Autodesk Inventor part; units mm, degrees
ref_plane "YZ Plane" through (0, 0, 0) normal (1, 0, 0) x (0, 1, 0)
ref_plane "XZ Plane" through (0, 0, 0) normal (0, 1, 0) x (-1, 0, 0)
ref_plane "XY Plane" through (0, 0, 0) normal (0, 0, 1) x (1, 0, 0)
sketch "Skizze1" plane through (0, 0, 0) normal (0, 0, 1) x (1, 0, 0)
  line L0 (25, 12.5) -> (-25, 12.5)
  line L1 (-25, 12.5) -> (-25, -12.5)
  line L2 (-25, -12.5) -> (25, -12.5)
  line L3 (25, -12.5) -> (25, 12.5)
  circle A0 centre (50.8, -8.2735) radius 14.6905
  circle A1 centre (50.8, -8.2735) radius 15
  line L4 (-63.7896, 27.9801) -> (95.321, 27.9801)
  line L5 (95.321, 27.9801) -> (95.321, -42.1521)
  line L6 (95.321, -42.1521) -> (-63.7896, -42.1521)
  line L7 (-63.7896, -42.1521) -> (-63.7896, 27.9801)
  point P0 (0, 0)
  dimension "d0" = 30
extrude "Extrusion1" add sketch "Skizze1" along normal blind 3 contours L4 L5 L6 L7
sketch "Skizze2" plane through (0, 0, 0) normal (0, 0, -1) x (-1, 0, 0)
  circle A0 centre (-50.8, -8.2735) radius 15 construction
  circle A1 centre (-50.8, -8.2735) radius 17.5
  point P0 (0, 0)
  dimension "d3" = 35
extrude "Extrusion2" cut sketch "Skizze2" against normal blind 1
sketch "Skizze3" plane through (0, 0, 0) normal (0, 0, -1) x (-1, 0, 0)
  circle A0 centre (-77.33, -20.3235) radius 1.75 construction
  circle A1 centre (40.52, -20.3235) radius 1.75 construction
  circle A2 centre (40.52, 8.5265) radius 1.75 construction
  circle A3 centre (-77.33, 8.5265) radius 1.75 construction
  arc A4 (-44.8513, -25.2196) -> (-44.1338, -24.9216) centre (-45.6338, -22.3235) ccw construction
  arc A5 (-44.8513, -25.2196) -> (-45.0539, -25.3294) centre (-44.7209, -25.7023) ccw construction
  arc A6 (-46.2827, -25.4102) -> (-45.0539, -25.3294) centre (-45.72, -24.5835) ccw construction
  arc A7 (-46.2827, -25.4102) -> (-46.564, -25.3235) centre (-46.564, -25.8235) ccw construction
  line L0 (-55.036, -25.3235) -> (-46.564, -25.3235) construction
  arc A8 (-55.036, -25.3235) -> (-55.3173, -25.4102) centre (-55.036, -25.8235) ccw construction
  arc A9 (-56.4427, -25.4102) -> (-55.3173, -25.4102) centre (-55.88, -24.5835) ccw construction
  arc A10 (-56.4427, -25.4102) -> (-56.724, -25.3235) centre (-56.724, -25.8235) ccw construction
  line L1 (-66.83, -25.3235) -> (-56.724, -25.3235) construction
  arc A11 (-67.83, -24.3235) -> (-66.83, -25.3235) centre (-66.83, -24.3235) ccw construction
  line L2 (-67.83, -14.2262) -> (-67.83, -24.3235) construction
  arc A12 (-67.83, -14.2262) -> (-67.9233, -13.9353) centre (-68.33, -14.2262) ccw construction
  arc A13 (-67.9233, -12.7717) -> (-67.9233, -13.9353) centre (-67.11, -13.3535) ccw construction
  arc A14 (-67.9233, -12.7717) -> (-67.83, -12.4808) centre (-68.33, -12.4808) ccw construction
  line L3 (-67.83, -4.0662) -> (-67.83, -12.4808) construction
  arc A15 (-67.83, -4.0662) -> (-67.9233, -3.7753) centre (-68.33, -4.0662) ccw construction
  arc A16 (-67.9233, -2.6117) -> (-67.9233, -3.7753) centre (-67.11, -3.1935) ccw construction
  arc A17 (-67.9233, -2.6117) -> (-67.83, -2.3208) centre (-68.33, -2.3208) ccw construction
  line L4 (-67.83, -1.6101) -> (-67.83, -2.3208) construction
  arc A18 (-67.83, -1.6101) -> (-68.1376, -1.1483) centre (-68.3305, -1.6101) ccw construction
  arc A19 (-68.445, -0.6869) -> (-68.1376, -1.1483) centre (-67.945, -0.6869) ccw construction
  line L5 (-68.445, 14.5865) -> (-68.445, -0.6869) construction
  arc A20 (-67.945, 15.0865) -> (-68.445, 14.5865) centre (-67.945, 14.5865) ccw construction
  line L6 (-58.801, 15.0865) -> (-67.945, 15.0865) construction
  arc A21 (-58.301, 14.5865) -> (-58.801, 15.0865) centre (-58.801, 14.5865) ccw construction
  line L7 (-58.301, 14.5265) -> (-58.301, 14.5865) construction
  arc A22 (-58.301, 14.5265) -> (-57.301, 13.5265) centre (-57.301, 14.5265) ccw construction
  line L8 (-44.045, 13.5265) -> (-57.301, 13.5265) construction
  arc A23 (-44.045, 13.5265) -> (-43.045, 14.5265) centre (-44.045, 14.5265) ccw construction
  line L9 (-43.045, 14.5865) -> (-43.045, 14.5265) construction
  arc A24 (-42.545, 15.0865) -> (-43.045, 14.5865) centre (-42.545, 14.5865) ccw construction
  line L10 (-33.401, 15.0865) -> (-42.545, 15.0865) construction
  arc A25 (-32.901, 14.5865) -> (-33.401, 15.0865) centre (-33.401, 14.5865) ccw construction
  line L11 (-32.901, 14.5265) -> (-32.901, 14.5865) construction
  arc A26 (-32.901, 14.5265) -> (-31.901, 13.5265) centre (-31.901, 14.5265) ccw construction
  line L12 (21.02, 13.5265) -> (-31.901, 13.5265) construction
  arc A27 (31.02, 3.5265) -> (21.02, 13.5265) centre (21.02, 3.5265) ccw construction
  line L13 (31.02, 2.4539) -> (31.02, 3.5265) construction
  arc A28 (31.02, 2.4539) -> (31.3225, 1.9945) centre (31.52, 2.4539) ccw construction
  arc A29 (31.3225, -0.7615) -> (31.3225, 1.9945) centre (30.73, 0.6165) ccw construction
  arc A30 (31.3225, -0.7615) -> (31.02, -1.2209) centre (31.52, -1.2209) ccw construction
  line L14 (31.02, -1.3561) -> (31.02, -1.2209) construction
  arc A31 (31.02, -1.3561) -> (31.3225, -1.8155) centre (31.52, -1.3561) ccw construction
  arc A32 (31.3225, -4.5715) -> (31.3225, -1.8155) centre (30.73, -3.1935) ccw construction
  arc A33 (31.3225, -4.5715) -> (31.02, -5.0309) centre (31.52, -5.0309) ccw construction
  line L15 (31.02, -5.1661) -> (31.02, -5.0309) construction
  arc A34 (31.02, -5.1661) -> (31.3225, -5.6255) centre (31.52, -5.1661) ccw construction
  arc A35 (31.3225, -8.3815) -> (31.3225, -5.6255) centre (30.73, -7.0035) ccw construction
  arc A36 (31.3225, -8.3815) -> (31.02, -8.8409) centre (31.52, -8.8409) ccw construction
  line L16 (31.02, -10.4303) -> (31.02, -8.8409) construction
  arc A37 (31.02, -10.4303) -> (31.3433, -10.898) centre (31.52, -10.4303) ccw construction
  arc A38 (31.3433, -12.769) -> (31.3433, -10.898) centre (30.99, -11.8335) ccw construction
  arc A39 (31.3433, -12.769) -> (31.02, -13.2367) centre (31.52, -13.2367) ccw construction
  line L17 (31.02, -20.5903) -> (31.02, -13.2367) construction
  arc A40 (31.02, -20.5903) -> (31.3433, -21.058) centre (31.52, -20.5903) ccw construction
  arc A41 (31.3283, -22.9345) -> (31.3433, -21.058) centre (30.99, -21.9935) ccw construction
  arc A42 (31.3283, -22.9345) -> (30.9977, -23.3898) centre (31.4974, -23.4051) ccw construction
  arc A43 (28.77, -25.3235) -> (30.9977, -23.3898) centre (28.77, -23.0735) ccw construction
  line L18 (-24.9736, -25.3235) -> (28.77, -25.3235) construction
  arc A44 (-26.4736, -24.9216) -> (-24.9736, -25.3235) centre (-24.9736, -22.3235) ccw construction
  line L19 (-33.8037, -20.6895) -> (-26.4736, -24.9216) construction
  arc A45 (-33.8037, -20.6895) -> (-36.8037, -20.6895) centre (-35.3037, -23.2876) ccw construction
  line L20 (-44.1338, -24.9216) -> (-36.8037, -20.6895) construction
  line L21 (-81.83, -30.3235) -> (45.02, -30.3235) construction
  arc A46 (45.02, -30.3235) -> (48.02, -27.3235) centre (45.02, -27.3235) ccw construction
  line L22 (48.02, -27.3235) -> (48.02, 15.5265) construction
  arc A47 (48.02, 15.5265) -> (45.02, 18.5265) centre (45.02, 15.5265) ccw construction
  line L23 (45.02, 18.5265) -> (-81.83, 18.5265) construction
  arc A48 (-81.83, 18.5265) -> (-84.83, 15.5265) centre (-81.83, 15.5265) ccw construction
  line L24 (-84.83, 15.5265) -> (-84.83, -27.3235) construction
  arc A49 (-84.83, -27.3235) -> (-81.83, -30.3235) centre (-81.83, -27.3235) ccw construction
  point P0 (0, 0)
hole "Bohrung1" at (77.33, 8.5265, 0) at (77.33, -20.3235, 0) at (-40.52, -20.3235, 0) at (-40.52, 8.5265, 0) direction (0, 0, 1) diameter 3 end through all
properties part number "Ausschnitt"
CAD build for the part. Positions are in the model's coordinates, mm. A direction names the side the tool comes from. Coordinates: 2 decimals unless noted, no trailing zeros. Write each loop counter-clockwise with the first axis right and the second up, starting at its lowest first coordinate (ties: lowest second). Pieces come first, ordered by that corner, then holes. Notation, with made-up numbers: (-8, 11) - (10, 11) arc R23 ccw to (10, 21) - close; hole circle Ø7 at (79, 46.5). An arc over 180 degrees is marked (long way). Use a Markdown table: item, result. Add a question column.
Item 1: Band-saw the part on B-B, the plane y = -1.5. Give the cut face in (x, z).
Item 2: Drill centre lines: L1, parallel to Y at x = -40.52, z = 2.35; L2, parallel to Y at x = 50.8, z = 2.65; L3, parallel to X at y = -2, z = 1.6. Where is each one in solid material? Low to high. Write a range as from..to.
Item 3: Band-saw the part on C-C, the plane x = -40.52. Give the cut face in (y, z), and give its area (3 significant figures).
Item 4: Band-saw the part on D-D, the plane z = 1.9. Give the cut face in (x, y), and give its area (3 significant figures).
Item 5: Mould opens along Y. For faces 1 (the face through (78.794, -20.649, 1.521)), 2 (the face through (17, -42.152, 1)), 3 (the face through (-63.79, -8, 1)) say: pulls with the +Y half, pulls with the -Y half, needs draft (parallel to the pull), parting line crosses it, or undercut.
Item 6: 3-axis set-ups, long thin cutter, end or side, ignore diameter. For faces 4 (the face through (68.283, -7.504, 0.493)), 5 (the face through (0, 12.5, 1)), 6 (the face through (15, -14, 0)): which of +Z, -Z, +X, -X, +Y, -Y reach the whole face in a straight line?
Item 7: Band-saw the part on A-A, the plane x = 50.8. Give the cut face in (y, z), and give its area (3 significant figures).
Numbers:
| question | item | result |
|---|---|---|
| 1 | outline | (-63.79, 0) - (-25, 0) - (-25, 3) - (-63.79, 3) - close; (25, 0) - (34.66, 0) - (34.66, 1) - (37.42, 1) - (37.42, 3) - (25, 3) - close; (64.18, 1) - (66.94, 1) - (66.94, 0) - (95.32, 0) - (95.32, 3) - (64.18, 3) - close |
| 2 | L1 | -42.15..-21.82, -18.82..7.03, 10.03..27.98 |
| 2 | L2 | -42.15..-23.27, 6.73..27.98 |
| 2 | L3 | -63.79..-25, 25..37.17, 64.43..95.32 |
| 3 | outline | (-42.15, 0) - (-21.82, 0) - (-21.82, 3) - (-42.15, 3) - close; (-18.82, 0) - (7.03, 0) - (7.03, 3) - (-18.82, 3) - close; (10.03, 0) - (27.98, 0) - (27.98, 3) - (10.03, 3) - close |
| 3 | area | 192 mm2 |
| 4 | outline | (-63.79, -42.15) - (95.32, -42.15) - (95.32, 27.98) - (-63.79, 27.98) - close; hole circle Ø3 at (-40.52, -20.32); hole circle Ø3 at (-40.52, 8.53); hole (-25, -12.5) - (25, -12.5) - (25, 12.5) - (-25, 12.5) - close; hole circle Ø30 at (50.8, -8.27); hole circle Ø3 at (77.33, -20.32); hole circle Ø3 at (77.33, 8.53) |
| 4 | area | 9,170 mm2 |
| 5 | face 1 | undercut |
| 5 | face 2 | pulls with the -Y half |
| 5 | face 3 | needs draft |
| 6 | face 4 | -Z |
| 6 | face 5 | +Z, -Z |
| 6 | face 6 | -Z, +X, -X, +Y, -Y |
| 7 | outline | (-42.15, 0) - (-25.77, 0) - (-25.77, 1) - (-23.27, 1) - (-23.27, 3) - (-42.15, 3) - close; (6.73, 1) - (9.23, 1) - (9.23, 0) - (27.98, 0) - (27.98, 3) - (6.73, 3) - close |
| 7 | area | 115 mm2 |
